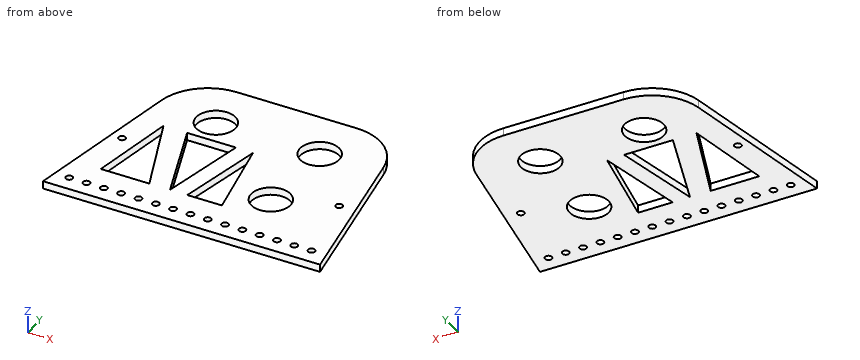
from build123d import *

# Parameters (mm, degrees)
SKETCH2_R           = 14.2875
SKETCH2_R_2         = 2.54
BOSS_EXTRUDE1_DEPTH = 5.55625
FILLET1_R           = 38.1


with BuildPart() as part:
    # Sketch2 → Boss-Extrude1 (new body)
    with BuildSketch(Plane.XY):
        Polygon((-33.221954044, -123.033671084), (-58.55568732, -123.033671084), (-33.221954044, 29.366328916), (119.178045956, 29.366328916), (144.745882617, -123.033671084), (119.178045956, -123.033671084), align=None)
        with Locations((4.878045956, -8.733671084)):
            Circle(SKETCH2_R, mode=Mode.SUBTRACT)
        with Locations((81.078045956, -8.733671084)):
            Circle(SKETCH2_R, mode=Mode.SUBTRACT)
        with Locations((-45.85568732, -111.187710863)):
            Circle(SKETCH2_R_2, mode=Mode.SUBTRACT)
        with Locations((-33.15568732, -111.187710863)):
            Circle(SKETCH2_R_2, mode=Mode.SUBTRACT)
        with Locations((-20.45568732, -111.187710863)):
            Circle(SKETCH2_R_2, mode=Mode.SUBTRACT)
        with Locations((-7.75568732, -111.187710863)):
            Circle(SKETCH2_R_2, mode=Mode.SUBTRACT)
        with Locations((4.94431268, -111.187710863)):
            Circle(SKETCH2_R_2, mode=Mode.SUBTRACT)
        with Locations((17.64431268, -111.187710863)):
            Circle(SKETCH2_R_2, mode=Mode.SUBTRACT)
        with Locations((30.34431268, -111.187710863)):
            Circle(SKETCH2_R_2, mode=Mode.SUBTRACT)
        with Locations((43.04431268, -111.187710863)):
            Circle(SKETCH2_R_2, mode=Mode.SUBTRACT)
        with Locations((55.74431268, -111.187710863)):
            Circle(SKETCH2_R_2, mode=Mode.SUBTRACT)
        with Locations((68.44431268, -111.187710863)):
            Circle(SKETCH2_R_2, mode=Mode.SUBTRACT)
        with Locations((81.14431268, -111.187710863)):
            Circle(SKETCH2_R_2, mode=Mode.SUBTRACT)
        with Locations((93.84431268, -111.187710863)):
            Circle(SKETCH2_R_2, mode=Mode.SUBTRACT)
        with Locations((106.54431268, -111.187710863)):
            Circle(SKETCH2_R_2, mode=Mode.SUBTRACT)
        with Locations((119.24431268, -111.187710863)):
            Circle(SKETCH2_R_2, mode=Mode.SUBTRACT)
        with Locations((131.94431268, -111.187710863)):
            Circle(SKETCH2_R_2, mode=Mode.SUBTRACT)
        with Locations((79.809453324, -71.051356873)):
            Circle(SKETCH2_R, mode=Mode.SUBTRACT)
        with Locations((121.810607633, -56.370137575)):
            Circle(SKETCH2_R_2, mode=Mode.SUBTRACT)
        with Locations((-38.87409027, -53.830137575)):
            Circle(SKETCH2_R_2, mode=Mode.SUBTRACT)
        Polygon((-22.767796965, -28.16783361), (-33.15568732, -92.394571291), (2.468038836, -92.394571291), align=None, mode=Mode.SUBTRACT)
        Polygon((43.04431268, -28.399699089), (55.74431268, -92.394571291), (30.34431268, -92.394571291), align=None, mode=Mode.SUBTRACT)
        Polygon((17.64431268, -92.394571291), (30.390327173, -28.16783361), (-5.41538745, -28.16783361), align=None, mode=Mode.SUBTRACT)
    extrude(amount=BOSS_EXTRUDE1_DEPTH)

    # Fillet1
    fillet1_edges = [part.edges().sort_by_distance(p)[0] for p in [
        (-33.221954044, 29.366328916, 2.778125),
        (119.178045956, 29.366328916, 2.778125),
    ]]
    fillet(fillet1_edges, radius=FILLET1_R)


solid = part.part
Design review of the part built by this model. Coordinates are the model's own, in mm. Coordinates: 2 decimals unless noted, no trailing zeros. Loops run counter-clockwise (first coordinate to the right, second up) from the corner with the lowest first, then second, coordinate; pieces in that order, holes last. Notation, with made-up numbers: (-37, 53.5) - (4, 53.5) arc R17 ccw to (4, 81.5) - close; hole circle Ø8 at (30, 50). An arc over 180 degrees is marked (long way). Use CSV: the item, a comma, the result in double quotes. Start each with the question number.
1. Add section D-D on z = 4.3. Count the separate pieces of the cut face and the enclosed holes in it, plus the area to 3 significant figures.
2. Add section A-A on x = -27.5. Give the boundary of the cut face in (y, z), plus the area to 3 significant figures.
3. Add section B-B on y = -38. Give the boundary of the cut face in (x, z), plus the area to 3 significant figures.
4. Add section C-C on y = -18. Give the boundary of the cut face in (x, z).
5. To check wall thickness, follow probe 1 along X at (y, z) = (-55.5, 3.25); probe 2 along X at (y, z) = (-45, 1.1); probe 3 along X at (y, z) = (-29, 0.8). State the ranges of each line that lie inside material, in increasing order.
Resolved:
1,separate pieces,"1"
1,enclosed holes,"23"
1,area,"21,300 mm2"
2,outline,"(-123.03, 0) - (-92.39, 0) - (-92.39, 5.56) - (-123.03, 5.56) - close; (-57.43, 0) - (18.58, 0) - (18.58, 5.56) - (-57.43, 5.56) - close"
2,area,"593 mm2"
3,outline,"(-44.42, 0) - (-24.36, 0) - (-24.36, 5.56) - (-44.42, 5.56) - close; (-18.9, 0) - (-1.89, 0) - (-1.89, 5.56) - (-18.9, 5.56) - close; (28.44, 0) - (41.14, 0) - (41.14, 5.56) - (28.44, 5.56) - close; (44.95, 0) - (130.48, 0) - (130.48, 5.56) - (44.95, 5.56) - close"
3,area,"752 mm2"
4,outline,"(-41.1, 0) - (-6, 0) - (-6, 5.56) - (-41.1, 5.56) - close; (15.75, 0) - (70.2, 0) - (70.2, 5.56) - (15.75, 5.56) - close; (91.95, 0) - (127.12, 0) - (127.12, 5.56) - (91.95, 5.56) - close"
5,probe 1,"-47.33 to -40.79, -36.96 to -27.19, -12.03 to 4.4, 24.97 to 37.67, 48.42 to 119.42, 124.2 to 133.42"
5,probe 2,"-45.58 to -25.49, -16.15 to 0.63, 27.05 to 39.75, 46.34 to 131.65"
5,probe 3,"-42.92 to -22.9, -22.44 to -5.12, 30.23 to 42.93, 43.16 to 128.97"
